Model file for the job. Use its own axes, mm. Coordinates: 2 decimals unless noted, no trailing zeros. Loops run counter-clockwise (first coordinate to the right, second up) from the corner with the lowest first, then second, coordinate; pieces in that order, holes last.
from build123d import *

# Parameters (mm, degrees)
SKETCH1_W           = 25.4
SKETCH1_H           = 25.4
SKETCH1_W_2         = 22.225
SKETCH1_H_2         = 22.225
BOSS_EXTRUDE1_DEPTH = 228.6
SKETCH2_R           = 2.0193
CUT_EXTRUDE1_DEPTH  = 26.4
SKETCH3_R           = 2.0193
CUT_EXTRUDE2_DEPTH  = 26.4


with BuildPart() as part:
    # Sketch1 → Boss-Extrude1 (new body)
    with BuildSketch(Plane(origin=(0, 0, 0), x_dir=(1, 0, 0), z_dir=(0, 1, 0))):
        with Locations((12.7, 12.7)):
            Rectangle(SKETCH1_W, SKETCH1_H)
        with Locations((12.7, 12.7)):
            Rectangle(SKETCH1_W_2, SKETCH1_H_2, mode=Mode.SUBTRACT)
    extrude(amount=BOSS_EXTRUDE1_DEPTH)

    # Sketch2 → Cut-Extrude1 (cut, through all)
    with BuildSketch(Plane.XY):
        with Locations((12.7, 12.7)):
            Circle(SKETCH2_R)
        with Locations((12.7, 25.4)):
            Circle(SKETCH2_R)
        with Locations((12.7, 38.1)):
            Circle(SKETCH2_R)
        with Locations((12.7, 50.8)):
            Circle(SKETCH2_R)
        with Locations((12.7, 63.5)):
            Circle(SKETCH2_R)
        with Locations((12.7, 76.2)):
            Circle(SKETCH2_R)
        with Locations((12.7, 88.9)):
            Circle(SKETCH2_R)
        with Locations((12.7, 101.6)):
            Circle(SKETCH2_R)
        with Locations((12.7, 114.3)):
            Circle(SKETCH2_R)
        with Locations((12.7, 127)):
            Circle(SKETCH2_R)
        with Locations((12.7, 139.7)):
            Circle(SKETCH2_R)
        with Locations((12.7, 152.4)):
            Circle(SKETCH2_R)
        with Locations((12.7, 165.1)):
            Circle(SKETCH2_R)
        with Locations((12.7, 177.8)):
            Circle(SKETCH2_R)
        with Locations((12.7, 190.5)):
            Circle(SKETCH2_R)
        with Locations((12.7, 203.2)):
            Circle(SKETCH2_R)
        with Locations((12.7, 215.9)):
            Circle(SKETCH2_R)
    extrude(amount=-CUT_EXTRUDE1_DEPTH, mode=Mode.SUBTRACT)

    # Sketch3 → Cut-Extrude2 (cut, through all)
    with BuildSketch(Plane(origin=(25.4, 0, 0), x_dir=(0, 0, -1), z_dir=(1, 0, 0))):
        with Locations((12.7, 12.7)):
            Circle(SKETCH3_R)
        with Locations((12.7, 25.4)):
            Circle(SKETCH3_R)
        with Locations((12.7, 38.1)):
            Circle(SKETCH3_R)
        with Locations((12.7, 50.8)):
            Circle(SKETCH3_R)
        with Locations((12.7, 63.5)):
            Circle(SKETCH3_R)
        with Locations((12.7, 76.2)):
            Circle(SKETCH3_R)
        with Locations((12.7, 88.9)):
            Circle(SKETCH3_R)
        with Locations((12.7, 101.6)):
            Circle(SKETCH3_R)
        with Locations((12.7, 114.3)):
            Circle(SKETCH3_R)
        with Locations((12.7, 127)):
            Circle(SKETCH3_R)
        with Locations((12.7, 139.7)):
            Circle(SKETCH3_R)
        with Locations((12.7, 152.4)):
            Circle(SKETCH3_R)
        with Locations((12.7, 165.1)):
            Circle(SKETCH3_R)
        with Locations((12.7, 177.8)):
            Circle(SKETCH3_R)
        with Locations((12.7, 190.5)):
            Circle(SKETCH3_R)
        with Locations((12.7, 203.2)):
            Circle(SKETCH3_R)
        with Locations((12.7, 215.9)):
            Circle(SKETCH3_R)
    extrude(amount=-CUT_EXTRUDE2_DEPTH, mode=Mode.SUBTRACT)


solid = part.part
Q1. Drill centre lines: line 1 (Z direction, x = 17.75, y = 107.5); line 2 (X direction, y = 108, z = -16); line 3 (X direction, y = 177.8, z = -0.8). Where is each one in solid material? Low to high.
Answers:
line 1: z = -25.4 to -23.81, -1.59 to 0
line 2: x = 0 to 1.59, 23.81 to 25.4
line 3: x = 0 to 10.68, 14.72 to 25.4
Q2. Mould opens along Z. For faces 1 (the cylindrical face through (0.8, 125.03, -12.26)), 2 (the flat face through (15, 113, -25.4)), 3 (the cylindrical face through (12.437, 52.802, -0.783)) say: +Z half, -Z half, draft (parallel to the pull), parting line (faces both ways), or undercut.
Answers:
face 1: undercut
face 2: -Z half
face 3: draft
Q3. Flat gauge pin, fed straight in: P1, Ø1.5, axis at x = 14, z = -23, coming from the -Y side. Where does the tip first touch, or does it go through?
Answers:
P1: passes through
Q4. Slice it at A-A (z = -5.5). List the corners of the cut face in (x, y), and give its area (3 significant figures).
Answers:
outline: (0, 0) - (1.59, 0) - (1.59, 228.6) - (0, 228.6) - close; (23.81, 0) - (25.4, 0) - (25.4, 228.6) - (23.81, 228.6) - close
area: 726 mm2
Q5. Slice it at B-B (y = 121.5). List the corners of the cut face in (x, z).
Answers:
outline: (0, -25.4) - (25.4, -25.4) - (25.4, 0) - (0, 0) - close; hole (1.59, -23.81) - (23.81, -23.81) - (23.81, -1.59) - (1.59, -1.59) - close
Q6. Slice it at C-C (x = 8). List the corners of the cut face in (y, z).
Answers:
outline: (0, -25.4) - (228.6, -25.4) - (228.6, -23.81) - (0, -23.81) - close; (0, -1.59) - (228.6, -1.59) - (228.6, 0) - (0, 0) - close
